The listing builds one solid part. Answer for the finished solid, in the listing's coordinates (mm). Round coordinates to 2 decimals unless told otherwise and drop trailing zeros. Loops run counter-clockwise (first coordinate to the right, second up) from the corner with the lowest first, then second, coordinate; pieces in that order, holes last. Notation, with made-up numbers: M -36,57.25 L -13,57.25 A19 ccw -13,79.25 Z; hole C 16,-15 d7. An arc over 180 degrees is marked long. Answer as a JSON object with one key per item and string values.
```python
from build123d import *

# Parameters (mm, degrees)
SKETCH1_W                    = 939.8
SKETCH1_H                    = 28.575
BASE_FLANGE1_DEPTH           = 3.175
EDGE_FLANGE1_STRIP_W         = 19.05
EDGE_FLANGE1_STRIP_H         = 3.175
EDGE_FLANGE1_STRIP_CUT_DEPTH = 939.8
EDGE_FLANGE1_DEPTH           = 939.8
F_11_0_191_DIAMETER_HOLE1_D  = 4.8514
LPATTERN1_COUNT              = 4
LPATTERN1_PITCH              = 304.8


# Sheet-metal steps are written as plain solids
with BuildPart() as part:
    # Sketch1 → Base-Flange1 (new body)
    with BuildSketch(Plane(origin=(0, 0, 0), x_dir=(1, 0, 0), z_dir=(0, 1, 0))):
        Rectangle(SKETCH1_W, SKETCH1_H)
    extrude(amount=-BASE_FLANGE1_DEPTH)

    # Edge-Flange1 strip (across the edge) → Edge-Flange1 strip cut (cut)
    with BuildSketch(Plane(origin=(469.9, 0, -14.2875), x_dir=(0, 0, 1), z_dir=(-1, 0, 0))):
        with Locations((-3.175, -1.5875)):
            Rectangle(EDGE_FLANGE1_STRIP_W, EDGE_FLANGE1_STRIP_H)
    extrude(amount=EDGE_FLANGE1_STRIP_CUT_DEPTH, mode=Mode.SUBTRACT)

    # Edge-Flange1 section (across the edge) → Edge-Flange1 (add)
    with BuildSketch(Plane(origin=(469.9, 0, -14.2875), x_dir=(0, 0, 1), z_dir=(-1, 0, 0))):
        with BuildLine():
            Line((0, 3.175), (0, 25.4))
            Line((0, 25.4), (3.175, 25.4))
            Line((3.175, 25.4), (3.175, 3.175))
            ThreePointArc((3.175, 3.175), (4.10493597, 0.92993597), (6.35, 0))
            Line((6.35, 0), (6.35, -3.175))
            ThreePointArc((6.35, -3.175), (1.859871939, -1.315128061), (0, 3.175))
        make_face()
    extrude(amount=EDGE_FLANGE1_DEPTH)

    # #11 (0.191) Diameter Hole1 (through all)
    with Locations(Plane(origin=(0, 0, 0), x_dir=(1, 0, 0), z_dir=(0, 1, 0))):
        with Locations((-457.2, 1.5875)):
            f_11_0_191_diameter_hole1 = Hole(F_11_0_191_DIAMETER_HOLE1_D / 2)

    # LPattern1: #11 (0.191) Diameter Hole1 ×4
    with Locations(*[(i * LPATTERN1_PITCH, 0, 0) for i in range(1, LPATTERN1_COUNT)]):
        add(f_11_0_191_diameter_hole1, mode=Mode.SUBTRACT)


solid = part.part
```
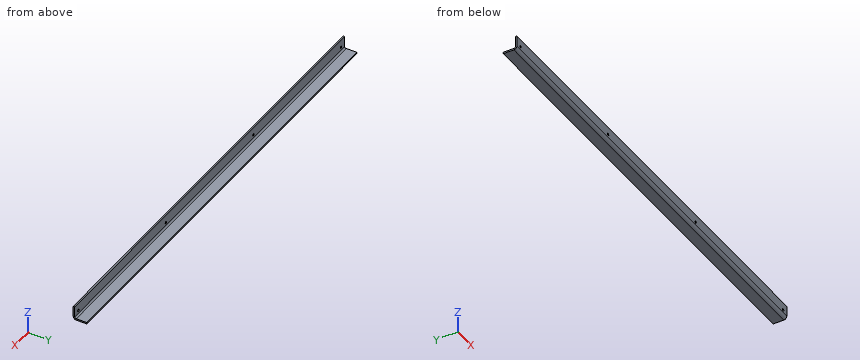
Item 1: Flat-ended cylindrical pins translate along their axes: P1, Ø8, axis at x = -152.4, z = -1.59, coming from the +Y side; P2, Ø5, axis at x = 254.5, z = -6, coming from the +Y side; P3, Ø4, axis at y = 6.5, z = -7.5, coming from the -X side; P4, Ø10, axis at x = 161.5, y = 1.5, coming from the +Z side. Find the tip coordinate at first contact, or state that the pin passes through.
Values follow:
{"P1": "y = 0", "P2": "y = 0.05", "P3": "through", "P4": "z = 14.29"}
Item 2: The part is cut by section B-B (y = 20.25). Give the vertices of the cut face in (x, z).
Values follow:
{"outline": "M -469.9,-14.29 L 469.9,-14.29 L 469.9,-11.11 L -469.9,-11.11 Z"}
Item 3: Straight lines are drawn through the part: line 1 (X direction, y = -0.25, z = 0); line 2 (Y direction, x = -417, z = -6.5) (3 decimals); line 3 (Z direction, x = 285.5, y = 16.75). For each, find the intervals that lie inside material, in ascending order.
Values follow:
{"line 1": "-469.9 to -459.03, -455.37 to -154.23, -150.57 to 150.57, 154.23 to 455.37, 459.03 to 469.9", "line 2": "-3.175 to 0", "line 3": "-14.29 to -11.11"}
